Could you check a few things on this model? Use its own coordinates, in mm. Face numbers are marked on the shaded views. A direction names the side the tool comes from. Round coordinates to 2 decimals unless told otherwise and drop trailing zeros. Loops run counter-clockwise (first coordinate to the right, second up) from the corner with the lowest first, then second, coordinate; pieces in that order, holes last. Notation, with made-up numbers: (-33.75, 76.25) -> (-14.75, 76.25) arc R23 ccw to (-14.75, 95.25) -> close; hole circle Ø8 at (-1, -24). An arc over 180 degrees is marked (long way). One line per item, written item: value.
from build123d import *

# Parameters (mm, degrees)
PAD_DEPTH                = 8.5
PAD001_DEPTH             = 2
PAD002_DEPTH             = 8.5
SKETCH003_W              = 2
SKETCH003_H              = 10
SKETCH003_W_2            = 14
SKETCH003_H_2            = 2
PAD003_DEPTH             = 8
SKETCH003_MIRRORED_2_W   = 2
SKETCH003_MIRRORED_2_H   = 10
SKETCH003_MIRRORED_2_W_2 = 14
SKETCH003_MIRRORED_2_H_2 = 2
PAD003_MIRRORED_2_DEPTH  = 8
PAD002_MIRRORED_2_DEPTH  = 8.5
PAD001_MIRRORED_2_DEPTH  = 2
PAD_MIRRORED_2_DEPTH     = 8.5


with BuildPart() as part:
    # Sketch → Pad (new body)
    with BuildSketch(Plane.XY):
        with BuildLine():
            ThreePointArc((18.2, 0), (15.643074, 9.302378), (8.690742, 15.990966))
            Line((8.690742, 15.990966), (7.5, 13.8))
            Line((0, 13.8), (7.5, 13.8))
            Line((0, 11.8), (0, 13.8))
            Line((8.504147, 11.8), (0, 11.8))
            Line((9.471711, 13.142552), (8.504147, 11.8))
            ThreePointArc((16.2, 0), (14.420155, 7.382353), (9.471711, 13.142552))
            Line((16.2, 0), (18.2, 0))
        make_face()
    pad = extrude(amount=PAD_DEPTH)

    # Sketch001 → Pad001 (join)
    with BuildSketch(Plane.XY):
        with BuildLine():
            ThreePointArc((18, 0), (15.499386, 9.152543), (8.692328, 15.762088))
            Line((8.692328, 15.762088), (7.5, 13.6))
            Line((0, 13.6), (7.5, 13.6))
            Line((0, 4), (0, 13.6))
            ThreePointArc((4, 0), (2.828427, 2.828427), (0, 4))
            Line((4, 0), (18, 0))
        make_face()
    pad001 = extrude(amount=PAD001_DEPTH)

    # Sketch002 → Pad002 (join)
    with BuildSketch(Plane.XY):
        with BuildLine():
            ThreePointArc((3.2, 0), (2.900626, 1.351432), (2.058519, 2.45))
            Line((2.058519, 2.45), (0, 2.45))
            Line((0, 2.45), (0, 4.45))
            Line((0, 4.45), (2.69026, 4.45))
            ThreePointArc((5.2, 0), (4.529313, 2.554471), (2.69026, 4.45))
            Line((3.2, 0), (5.2, 0))
        make_face()
    pad002 = extrude(amount=PAD002_DEPTH)

    # Sketch003 → Pad003 (join)
    with BuildSketch(Plane.XY):
        with Locations((1, 9)):
            Rectangle(SKETCH003_W, SKETCH003_H)
        with Locations((11, 1)):
            Rectangle(SKETCH003_W_2, SKETCH003_H_2)
    pad003 = extrude(amount=PAD003_DEPTH)

    # Sketch003 Mirrored 2 → Pad003 Mirrored 2 (add)
    with BuildSketch(Plane(origin=(0, 0, 0), x_dir=(-1, 0, 0), z_dir=(0, 0, -1))):
        with Locations((1, 9)):
            Rectangle(SKETCH003_MIRRORED_2_W, SKETCH003_MIRRORED_2_H)
        with Locations((11, 1)):
            Rectangle(SKETCH003_MIRRORED_2_W_2, SKETCH003_MIRRORED_2_H_2)
    pad003_mirrored_2 = extrude(amount=-PAD003_MIRRORED_2_DEPTH)

    # Sketch002 Mirrored 2 → Pad002 Mirrored 2 (add)
    with BuildSketch(Plane(origin=(0, 0, 0), x_dir=(-1, 0, 0), z_dir=(0, 0, -1))):
        with BuildLine():
            ThreePointArc((3.2, 0), (2.900626, 1.351432), (2.058519, 2.45))
            Line((2.058519, 2.45), (0, 2.45))
            Line((0, 2.45), (0, 4.45))
            Line((0, 4.45), (2.69026, 4.45))
            ThreePointArc((5.2, 0), (4.529313, 2.554471), (2.69026, 4.45))
            Line((3.2, 0), (5.2, 0))
        make_face()
    pad002_mirrored_2 = extrude(amount=-PAD002_MIRRORED_2_DEPTH)

    # Sketch001 Mirrored 2 → Pad001 Mirrored 2 (add)
    with BuildSketch(Plane(origin=(0, 0, 0), x_dir=(-1, 0, 0), z_dir=(0, 0, -1))):
        with BuildLine():
            ThreePointArc((18, 0), (15.499386, 9.152543), (8.692328, 15.762088))
            Line((8.692328, 15.762088), (7.5, 13.6))
            Line((0, 13.6), (7.5, 13.6))
            Line((0, 4), (0, 13.6))
            ThreePointArc((4, 0), (2.828427, 2.828427), (0, 4))
            Line((4, 0), (18, 0))
        make_face()
    pad001_mirrored_2 = extrude(amount=-PAD001_MIRRORED_2_DEPTH)

    # Sketch Mirrored 2 → Pad Mirrored 2 (add)
    with BuildSketch(Plane(origin=(0, 0, 0), x_dir=(-1, 0, 0), z_dir=(0, 0, -1))):
        with BuildLine():
            ThreePointArc((18.2, 0), (15.643074, 9.302378), (8.690742, 15.990966))
            Line((8.690742, 15.990966), (7.5, 13.8))
            Line((0, 13.8), (7.5, 13.8))
            Line((0, 11.8), (0, 13.8))
            Line((8.504147, 11.8), (0, 11.8))
            Line((9.471711, 13.142552), (8.504147, 11.8))
            ThreePointArc((16.2, 0), (14.420155, 7.382353), (9.471711, 13.142552))
            Line((16.2, 0), (18.2, 0))
        make_face()
    pad_mirrored_2 = extrude(amount=-PAD_MIRRORED_2_DEPTH)

    # Mirrored001: Pad003, Pad002, Pad001, Pad, Pad003 Mirrored 2, Pad002 Mirrored 2, Pad001 Mirrored 2, Pad Mirrored 2 across Sketch003 H_Axis
    add(pad003.mirror(Plane.ZX))
    add(pad002.mirror(Plane.ZX))
    add(pad001.mirror(Plane.ZX))
    add(pad.mirror(Plane.ZX))
    add(pad003_mirrored_2.mirror(Plane.ZX))
    add(pad002_mirrored_2.mirror(Plane.ZX))
    add(pad001_mirrored_2.mirror(Plane.ZX))
    add(pad_mirrored_2.mirror(Plane.ZX))


solid = part.part
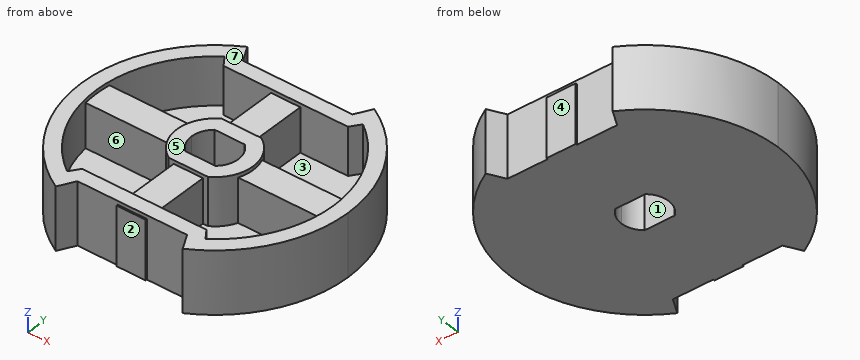
(1) If we section it at C-C, the plane y = 14.5: Please give me the cut outline in (x, z), then the cut area to 3 significant figures.
Recorded:
outline: (-11, 0) -> (-7.88, 0) -> (-7.88, 8.5) -> (-11, 8.5) -> close; (7.88, 0) -> (11, 0) -> (11, 8.5) -> (7.88, 8.5) -> close
area: 53.0 mm²
(2) For the marked faces 1, 2, 3, 4 and 5, which set-ups out of +Z, -Z, +X, -X, +Y, -Y let a thin tool reach every point of the face, with its end or its side?
Recorded:
face 1: +Z, -Z
face 2: +Z, -Z, -Y
face 3: +Z
face 4: +Z, -Z, +Y
face 5: +Z, +X, -X, +Y, -Y
(3) If we section it at D-D, the plane x = 15: Please give me the cut outline in (y, z), then the cut area to 3 significant figures.
Recorded:
outline: (-10.31, 0) -> (10.31, 0) -> (10.31, 8.5) -> (6.12, 8.5) -> (6.12, 2) -> (2, 2) -> (2, 8) -> (-2, 8) -> (-2, 2) -> (-6.12, 2) -> (-6.12, 8.5) -> (-10.31, 8.5) -> close
area: 120 mm²
(4) Thinking about a two-plate mould opening in X: for the marked faces 6 and 7, which applies, released by +X, released by -X, zero draft, split by the parting line, or undercut?
Recorded:
face 6: undercut
face 7: zero draft
(5) If I drill on L1, parallel to Y at x = -2.5, z = 3; L2, parallel to Y at x = 6, z = 5.75; L3, parallel to X at y = -5, z = 5.25, over which ranges is the centre line in solid material (lowest first)?
Recorded:
L1: -13.8 to -11.8, -4.45 to -2, 2 to 4.45, 11.8 to 13.8
L2: -13.8 to -11.8, -2 to 2, 11.8 to 13.8
L3: -17.5 to -15.41, -2 to 2, 15.41 to 17.5
(6) If we section it at B-B, the plane z = 1.25: Please give me the cut outline in (x, y), then the cut area to 3 significant figures.
Recorded:
outline: (-8.69, -15.99) -> (-7.5, -13.8) -> (-2, -13.8) -> (-2, -14) -> (2, -14) -> (2, -13.8) -> (7.5, -13.8) -> (8.69, -15.99) arc R18.2 ccw to (8.69, 15.99) -> (7.5, 13.8) -> (2, 13.8) -> (2, 14) -> (-2, 14) -> (-2, 13.8) -> (-7.5, 13.8) -> (-8.69, 15.99) arc R18.2 ccw to start; hole (-2.06, -2.45) -> (2.06, -2.45) arc R3.2 ccw to (2.06, 2.45) -> (-2.06, 2.45) arc R3.2 ccw to start
area: 891 mm²
(7) If we section it at A-A, the plane x = 1.5: Please give me the cut outline in (y, z).
Recorded:
outline: (-14, 0) -> (-2.45, 0) -> (-2.45, 8.5) -> (-4.45, 8.5) -> (-4.45, 8) -> (-11.8, 8) -> (-11.8, 8.5) -> (-13.8, 8.5) -> (-13.8, 8) -> (-14, 8) -> close; (2.45, 0) -> (14, 0) -> (14, 8) -> (13.8, 8) -> (13.8, 8.5) -> (11.8, 8.5) -> (11.8, 8) -> (4.45, 8) -> (4.45, 8.5) -> (2.45, 8.5) -> close
(8) I'm going to push flat-ended pins straight in: pin 1 Ø4.5 at (x, y) = (-11.5, 0.5) entering from +Z; pin 2 Ø2 at (x, z) = (0, 4) entering from +Y; pin 3 Ø3.5 at (x, y) = (-9, 10) entering from +Z. Where does each tip first touch, or does it pass through?
Recorded:
pin 1: z = 8
pin 2: y = 14
pin 3: z = 2
